Could you check a few things on this model? Use its own coordinates, in mm. Round coordinates to 2 decimals unless told otherwise and drop trailing zeros. Loops run counter-clockwise (first coordinate to the right, second up) from the corner with the lowest first, then second, coordinate; pieces in that order, holes last. Notation, with made-up numbers: (69, -30) -> (73, -30) arc R33 cw to (73, 9) -> close; hole circle Ø10 at (-23.5, 40.25). An arc over 180 degrees is marked (long way). One line per item, written item: value.
from build123d import *

# Parameters (mm, degrees)
F1_DEPTH = 20
F3_D     = 5
F3_DEPTH = 10
F3_TIP   = 1.5021515476
F5_D     = 5
F5_DEPTH = 10
F5_TIP   = 1.5021515476


with BuildPart() as f1:
    # F0 (on Top) → F1 (new body)
    with BuildSketch(Plane.XY):
        Polygon((-100, 0), (0, 0), (0, 100), align=None)
    extrude(amount=F1_DEPTH)

    # F3
    with Locations(Plane.YZ):
        with Locations((75, 10), (25, 10)):
            Hole(F3_D / 2, depth=F3_DEPTH)
            with Locations((0, 0, -(F3_DEPTH + F3_TIP / 2))):  # 118° drill point
                Cone(0, F3_D / 2, F3_TIP, mode=Mode.SUBTRACT)

    # F5
    with Locations(Plane.XZ):
        with Locations((-25, 10), (-75, 10)):
            Hole(F5_D / 2, depth=F5_DEPTH)
            with Locations((0, 0, -(F5_DEPTH + F5_TIP / 2))):  # 118° drill point
                Cone(0, F5_D / 2, F5_TIP, mode=Mode.SUBTRACT)


solid = f1.part
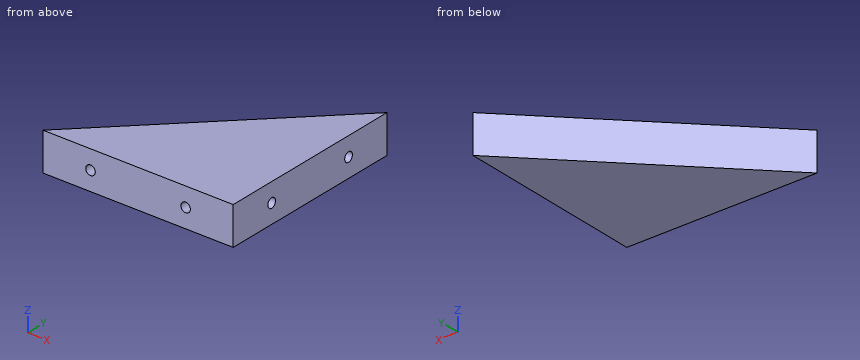
(1) If we section it at A-A, the plane y = 67.5: Please give me the cut outline in (x, z).
Recorded:
outline: (-32.5, 0) -> (0, 0) -> (0, 20) -> (-32.5, 20) -> close
(2) If we section it at B-B, the plane x = -52: Please give me the cut outline in (y, z), then the cut area to 3 significant figures.
Recorded:
outline: (0, 0) -> (48, 0) -> (48, 20) -> (0, 20) -> close
area: 960 mm²
(3) I'm going to push flat-ended pins straight in: pin 1 Ø4 at (x, z) = (-25, 10) entering from -Y; pin 2 Ø12 at (y, z) = (82.5, 12.5) entering from -X; pin 3 Ø4.5 at (y, z) = (25, 10) entering from +X; pin 4 Ø5 at (x, z) = (-80.5, 14) entering from -Y. Where does each tip first touch, or does it pass through?
Recorded:
pin 1: y = 10.3
pin 2: x = -23.5
pin 3: x = -10.15
pin 4: y = 0
(4) If I drill on L1, parallel to Z at x = -5, y = 25; L2, parallel to Y at x = -3.5, z = 10; L3, parallel to Y at x = -27.5, z = 3, over which ranges is the centre line in solid material (lowest first)?
Recorded:
L1: 0 to 7.5, 12.5 to 20
L2: 0 to 22.5, 27.5 to 72.5, 77.5 to 96.5
L3: 0 to 72.5
(5) If we section it at C-C, the plane z = 2.5: Please give me the cut outline in (x, y).
Recorded:
outline: (-100, 0) -> (0, 0) -> (0, 100) -> close
